CAD build for the part. Positions are in the model's coordinates, mm. A direction names the side the tool comes from. Round coordinates to 2 decimals unless told otherwise and drop trailing zeros. Order: outer loops, then holes, each group sorted by start corner. A loop starts at its lowest first (then second) coordinate and runs counter-clockwise, first axis right, second up. Notation, with made-up numbers: M 7.5,5 L 13.5,5 A17 cw 13.5,16 Z; hole C 73,54.25 d4. An arc over 180 degrees is marked long. Answer as a JSON object with one key per item and string values. Group by question number.
Autodesk Inventor part; units mm, degrees
ref_plane "YZ Plane" through (0, 0, 0) normal (1, 0, 0) x (0, 1, 0)
ref_plane "XZ Plane" through (0, 0, 0) normal (0, 1, 0) x (-1, 0, 0)
ref_plane "XY Plane" through (0, 0, 0) normal (0, 0, 1) x (1, 0, 0)
sketch "スケッチ1" plane through (0, 0, 0) normal (0, 1, 0) x (-1, 0, 0)
  line L0 (4.4873, 36.645) -> (-3.5127, 36.645)
  line L1 (-3.5127, 36.645) -> (-3.5127, -15.255)
  line L2 (-3.5127, -15.255) -> (4.4873, -15.255)
  line L3 (4.4873, -15.255) -> (4.4873, 36.645)
  circle A0 centre (0.4873, -12.255) radius 2.5
  line L4 (4.4873, 36.645) -> (9.3325, 36.645)
  line L5 (9.3325, 36.645) -> (9.3325, 26.645)
  line L6 (9.3325, 26.645) -> (4.4873, 26.645)
  line L7 (4.4873, 26.645) -> (4.4873, 36.645)
  point P0 (0, 0)
  dimension "d0" = 5
  dimension "d1" = 3
  dimension "d2" = 4
  dimension "d3" = 4
  dimension "d4" = 46.4
  dimension "d5" = 10
extrude "押し出し1" add sketch "スケッチ1" against normal blind 3 contours L3 L2 L1 L0
sketch "スケッチ2" plane through (0, 0, 0) normal (0, 1, 0) x (1, 0, 0)
  line L0 (3.5127, -36.645) -> (-4.4873, -36.645)
  line L1 (3.5127, 15.255) -> (3.5127, -36.645)
  line L2 (-4.4873, -36.645) -> (3.5127, -36.645)
  line L3 (3.5127, -36.645) -> (3.5127, 15.255)
  line L4 (3.5127, 15.255) -> (-4.4873, 15.255)
  line L5 (-4.4873, 15.255) -> (-4.4873, -36.645)
  circle A0 centre (-0.4873, 12.255) radius 1.5
  circle A1 centre (-0.4873, 12.255) radius 2.5
  point P0 (0, 0)
  dimension "d8" = 3
extrude "押し出し2" add sketch "スケッチ2" along normal blind 1 contours L0 L5 L4 L1 | A1
sketch "スケッチ3" plane through (0, -3, 0) normal (0, -1, 0) x (1, 0, 0)
  line L0 (-4.4873, 36.645) -> (-4.4873, -15.255)
  line L1 (-4.4873, 36.645) -> (-6.4873, 36.645)
  line L2 (-6.4873, 36.645) -> (-6.4873, 26.645)
  line L3 (-6.4873, 26.645) -> (-4.4873, 26.645)
  line L4 (-4.4873, 26.645) -> (-4.4873, 36.645)
  line L5 (-4.4873, 36.645) -> (3.5127, 36.645)
  line L6 (3.5127, 36.645) -> (3.5127, 9.2999)
  line L7 (3.5127, 9.2999) -> (-4.4873, 9.2999)
  line L8 (-4.4873, 9.2999) -> (-4.4873, 36.645)
  line L9 (3.5127, -15.255) -> (3.5127, 36.645)
  point P0 (0, 0)
  dimension "d11" = 10
  dimension "d12" = 0
  dimension "d24" = 2
extrude "押し出し3" add sketch "スケッチ3" along normal blind 16.6
chamfer "面取り1" distance 7 angle 45 1 edges at (3.5127, -9.3, 36.645)
chamfer "面取り3" distance 15 distance2 6.8 1 edges at (-4.9873, -19.6, 36.645) measured on face at (0.846, -19.6, 21.8633)
sketch "スケッチ4" plane through (0, 1, 0) normal (0, 1, 0) x (1, 0, 0)
  line L0 (-4.4873, -36.645) -> (-6.4873, -36.645)
  line L1 (3.5127, -9.2999) -> (-4.4873, -9.2999)
  line L2 (-6.4873, -36.645) -> (3.5127, -36.645)
  line L3 (3.5127, -36.645) -> (3.5127, -9.2999)
  line L4 (3.5127, -9.2999) -> (-6.4873, -9.2999)
  line L5 (-6.4873, -9.2999) -> (-6.4873, -36.645)
  point P0 (0, 0)
extrude "押し出し4" cut sketch "スケッチ4" against normal blind 4
chamfer "面取り4" distance 6.8 distance2 15 1 edges at (-4.9873, -3, 36.645) measured on face at (-4.4873, -9.5333, 36.645)
sketch "スケッチ5" plane through (0, -3, 0) normal (0, 1, 0) x (1, 0, 0)
  line L0 (3.5127, -21.645) -> (-4.4873, -21.645)
  line L1 (-4.4873, -9.2999) -> (-4.4873, 15.255)
  line L2 (3.5127, -21.645) -> (-4.4873, -21.645)
  line L3 (-4.4873, -21.645) -> (-4.4873, -9.2999)
  line L4 (-4.4873, -9.2999) -> (3.5127, -9.2999)
  line L5 (3.5127, -9.2999) -> (3.5127, -21.645)
  point P0 (0, 0)
extrude "押し出し5" add sketch "スケッチ5" along normal blind 4
properties part number "armmodulepart2"
Item 1: Cut at B-B, the plane y = -7.5. Give the cut face in (x, z) (3 decimals), and give its area (3 significant figures).
Item 2: Flat gauge pins, fed straight in: pin 1 Ø10 at (y, z) = (-12.5, -4) entering from -X; pin 2 Ø1.5 at (x, y) = (-2.5, -3) entering from +Z; pin 3 Ø6 at (x, y) = (-1, -9) entering from -Z; pin 4 Ø5.5 at (x, z) = (-0.5, -13) entering from -Y. Where does each tip first touch, or does it go through?
Item 3: Cut at C-C, the plane z = 12.5. Give the cut face in (x, y), and give its area (3 significant figures).
Item 4: Cut at A-A, the plane x = 0. Give the cut face in (y, z) (3 decimals), and give its area (3 significant figures).
Item 5: Two-plate mould, pull along Z, no slides. Class faces 1 (the face through (-0.683, 0.493, -10.768)), 2 (the face through (0, -3, -3)), 3 (the face through (0.84, -11.23, 32.32)): +Z half, -Z half, draft (parallel to the pull), parting line (faces both ways), or undercut.
Item 6: Drill centre lines: line 1 (Z direction, x = -3.5, y = -0.5) (3 decimals); line 2 (X direction, y = -3.5, z = 15.5); line 3 (Y direction, x = 3.25, z = 6). Where is each one in solid material? Low to high. Write a range as [from, to].
Item 7: Cut at D-D, the plane y = -1.25. Give the cut face in (x, z) (3 decimals), and give its area (3 significant figures).
Item 8: 3-axis set-ups, long thin cutter, end or side, ignore diameter. For faces 4 (the face through (0.055, -1.479, -14.696)), 5 (the face through (0, -11, 9.3)), 6 (the face through (0, -1, 21.645)): which of +Z, -Z, +X, -X, +Y, -Y reach the whole face in a straight line?
Response values:
{
 "1": {"outline": "M -6.487,26.645 L -4.487,26.645 L -4.487,9.3 L 3.513,9.3 L 3.513,29.645 L 1.586,31.571 L -6.487,31.571 Z", "area": "186 mm^2"},
 "2": {"pin 1": "through", "pin 2": "z = 23.3", "pin 3": "z = 9.3", "pin 4": "y = -3"},
 "3": {"outline": "M -4.49,-19.6 L 3.51,-19.6 L 3.51,1 L -4.49,1 Z", "area": "165 mm^2"},
 "4": {"outline": "M -19.6,9.3 L -3,9.3 L -3,-9.803 L 0,-9.803 L 0,-10.836 L 1,-10.836 L 1,21.645 L -3,21.645 L -8.219,33.158 L -14.381,33.158 L -19.6,21.645 Z; M -3,-15.255 L 1,-15.255 L 1,-13.674 L 0,-13.674 L 0,-14.707 L -3,-14.707 Z", "area": "466 mm^2"},
 "5": {"face 1": "undercut", "face 2": "draft", "face 3": "+Z half"},
 "6": {"line 1": "[-15.255, 21.645]", "line 2": "[-4.49, 3.51]", "line 3": "[-3, 1]"},
 "7": {"outline": "M -4.487,-15.255 L 3.513,-15.255 L 3.513,21.645 L -4.487,21.645 Z; hole C -0.487,-12.255 d5", "area": "276 mm^2"},
 "8": {"face 4": "-Y", "face 5": "-Z, +X, -X, -Y", "face 6": "+Z, +X, -X, +Y"}
}
